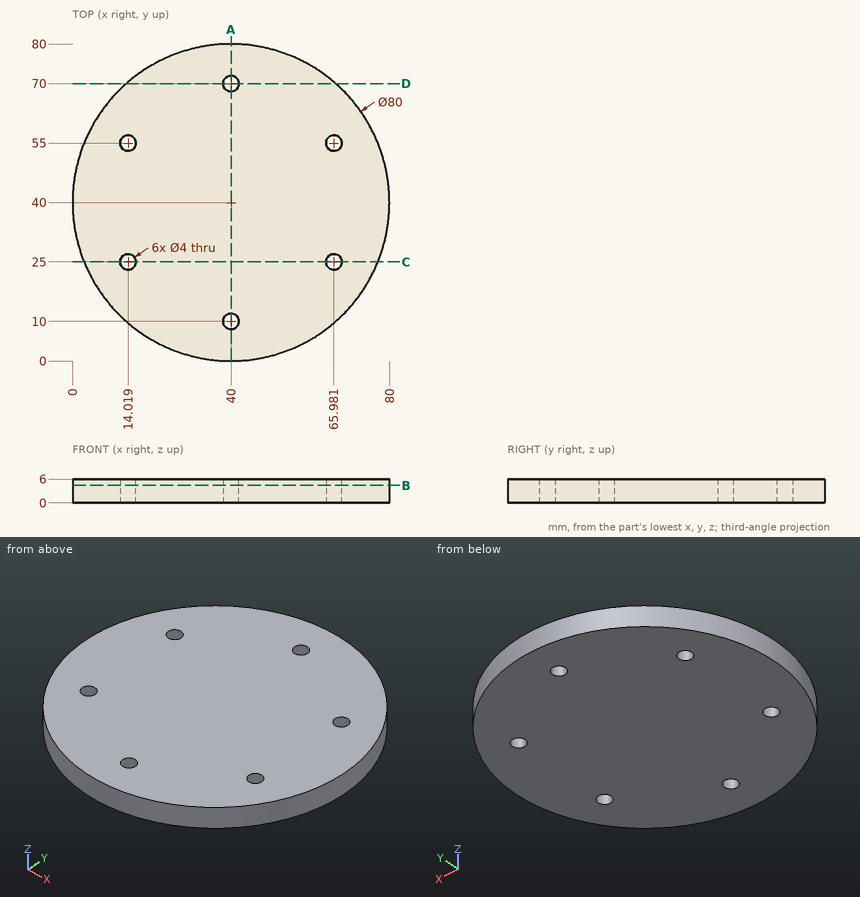
Could you check a few things on this drawing? It's one solid part, dimensions in mm from its lowest x, y, z. Round coordinates to 2 decimals unless told otherwise and drop trailing zeros. Loops run counter-clockwise (first coordinate to the right, second up) from the corner with the lowest first, then second, coordinate; pieces in that order, holes last. Notation, with made-up numbers: M 17.5,-31.5 L 22.5,-31.5 A24 ccw 22.5,-10.5 Z; hole C 6,53 d1. An arc over 180 degrees is marked long. Write item = value, one per line. Start each with the question number.
(1) Suppose I cut it at C-C on y = 25. Write out the boundary of the cut face in (x, z).
(2) Suppose I cut it at D-D on y = 70. Write out the boundary of the cut face in (x, z).
(3) Suppose I cut it at A-A on x = 40. Write out the boundary of the cut face in (y, z), plus the area to 3 significant figures.
(4) Suppose I cut it at B-B on z = 4.4. Write out the boundary of the cut face in (x, y), plus the area to 3 significant figures.
(5) I'm going to push flat-ended pins straight in: P1, Ø2, axis at x = 13.5, z = 2.5, coming from the +Y side; P2, Ø2, axis at x = 17.5, z = 2, coming from the -Y side. Where does each tip first touch, or does it pass through?
(6) I need wall thicknesses on line 1 along Y through (x, z) = (40, 1.25); line 2 along Y through (x, z) = (12.5, 5.25); line 3 along X through (y, z) = (55, 3.45). Which ranges of each line are inside material? Lowest first, please.
Answer block:
q1.outline = M 2.92,0 L 12.02,0 L 12.02,6 L 2.92,6 Z; M 16.02,0 L 63.98,0 L 63.98,6 L 16.02,6 Z; M 67.98,0 L 77.08,0 L 77.08,6 L 67.98,6 Z
q2.outline = M 13.54,0 L 38,0 L 38,6 L 13.54,6 Z; M 42,0 L 66.46,0 L 66.46,6 L 42,6 Z
q3.outline = M 0,0 L 8,0 L 8,6 L 0,6 Z; M 12,0 L 68,0 L 68,6 L 12,6 Z; M 72,0 L 80,0 L 80,6 L 72,6 Z
q3.area = 432 mm²
q4.outline = C 40,40 d80; hole C 14.02,25 d4; hole C 14.02,55 d4; hole C 40,10 d4; hole C 40,70 d4; hole C 65.98,25 d4; hole C 65.98,55 d4
q4.area = 4,950 mm²
q5.P1 = 70.82
q5.P2 = 6.27
q6.line_1 = 0 to 8, 12 to 68, 72 to 80
q6.line_2 = 10.95 to 23.7, 26.3 to 53.7, 56.3 to 69.05
q6.line_3 = 2.92 to 12.02, 16.02 to 63.98, 67.98 to 77.08
